The listing builds one solid part. Answer for the finished solid, in the listing's coordinates (mm). Face numbers are marked on the shaded views. Give positions to 0.01 mm unless a question says otherwise; leave off trailing zeros. Order: outer loops, then holes, each group sorted by start corner. A loop starts at its lowest first (then second) coordinate and runs counter-clockwise, first axis right, second up. Notation, with made-up numbers: (58, 69) - (96, 69) arc R18 ccw to (96, 82) - close; hole circle Ø11 at (-33.75, 68). An arc over 180 degrees is marked (long way). Answer in a Markdown table with one row per item.
from build123d import *

# Parameters (mm, degrees)
SKETCH1_W                        = 101.6
SKETCH1_H                        = 19.05
EXTRUDE1_DEPTH                   = 4.7625
F_39_64_0_60938_DIAMETER_HOLE1_D = 15.478252
F_1_4_0_25_DIAMETER_HOLE1_D      = 6.35
F_8_0_199_DIAMETER_HOLE1_D       = 5.0546


with BuildPart() as part:
    # Sketch1 → Extrude1 (new body)
    with BuildSketch(Plane(origin=(0, 0, 0), x_dir=(1, 0, 0), z_dir=(0, 1, 0))):
        Rectangle(SKETCH1_W, SKETCH1_H)
    extrude(amount=EXTRUDE1_DEPTH)

    # 39/64 (0.60938) Diameter Hole1 (through all)
    with Locations(Plane(origin=(0, 4.7625, 0), x_dir=(-1, 0, 0), z_dir=(0, 1, 0))):
        with Locations((25.4, 0), (-25.4, 0)):
            Hole(F_39_64_0_60938_DIAMETER_HOLE1_D / 2)

    # 1/4 (0.25) Diameter Hole1 (through all)
    with Locations(Plane.XY.offset(9.525)):
        with Locations((0, 4.7625), (-13.462, 4.7625), (13.462, 4.7625), (-38.481, 4.7625), (38.481, 4.7625)):
            Hole(F_1_4_0_25_DIAMETER_HOLE1_D / 2)

    # #8 (0.199) Diameter Hole1 (through all)
    with Locations(Plane(origin=(0, 4.7625, 0), x_dir=(-1, 0, 0), z_dir=(0, 1, 0))):
        with Locations((-46.228, 0), (-6.731, 0), (6.731, 0), (46.228, 0)):
            Hole(F_8_0_199_DIAMETER_HOLE1_D / 2)


solid = part.part
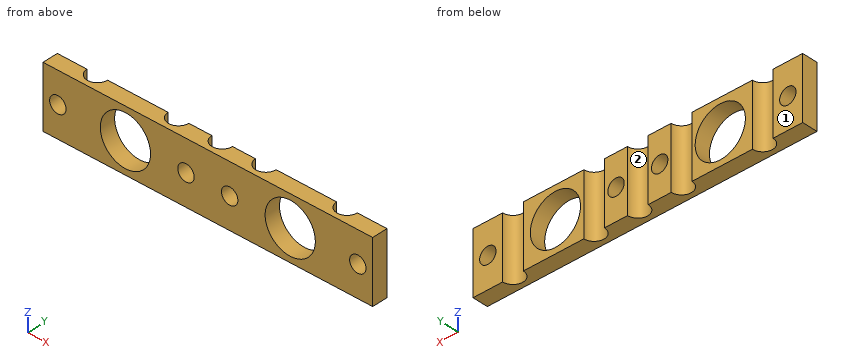
Item 1: Consider line 1 (X direction, y = 0.7, z = -3.5); line 2 (X direction, y = 0.8, z = -5); line 3 (Z direction, x = -18.5, y = 1.1) (3 decimals). Determine where each line is inside the solid, lowest interval first.
Answer block:
| item | result |
|---|---|
| line 1 | -50.8 to -32.3, -18.5 to 18.5, 32.3 to 50.8 |
| line 2 | -50.8 to -31.31, -19.49 to 19.49, 31.31 to 50.8 |
| line 3 | -9.525 to -3.505, 3.505 to 9.525 |
Item 2: Determine the mould class of the marked faces 1 and 2 for opening direction X: pulls with the +X half, pulls with the -X half, needs draft (parallel to the pull), parting line crosses it, or undercut.
Answer block:
| item | result |
|---|---|
| face 1 | needs draft |
| face 2 | undercut |
Item 3: Find section A-A on x = -25.4. Write down the section's boundary in (y, z) (1 decimal).
Answer block:
| item | result |
|---|---|
| outline | (0, -9.5) - (4.8, -9.5) - (4.8, -7.7) - (0, -7.7) - close; (0, 7.7) - (4.8, 7.7) - (4.8, 9.5) - (0, 9.5) - close |
Item 4: Find section B-B on z = -3.75. Count the separate pieces of the cut face and the enclosed holes in it, then the cut area to 3 significant figures.
Answer block:
| item | result |
|---|---|
| separate pieces | 3 |
| enclosed holes | 0 |
| area | 276 mm² |
